```python
from build123d import *

# Parameters (mm, degrees)
SKETCH1_W           = 200
SKETCH1_H           = 70
BOSS_EXTRUDE1_DEPTH = 10
SKETCH2_W           = 200
SKETCH2_H           = 20
BOSS_EXTRUDE2_DEPTH = 30
SKETCH3_W           = 200
SKETCH3_H           = 20
BOSS_EXTRUDE3_DEPTH = 30
SKETCH4_R           = 12.5
CUT_EXTRUDE1_DEPTH  = 30
SKETCH5_W           = 50
SKETCH5_H           = 50
CUT_EXTRUDE2_DEPTH  = 30


with BuildPart() as part:
    # Sketch1 → Boss-Extrude1 (new body)
    with BuildSketch(Plane(origin=(0, 0, 0), x_dir=(1, 0, 0), z_dir=(0, 1, 0))):
        with Locations((-100, 35)):
            Rectangle(SKETCH1_W, SKETCH1_H)
    extrude(amount=BOSS_EXTRUDE1_DEPTH)

    # Sketch2 → Boss-Extrude2 (add)
    with BuildSketch(Plane(origin=(0, 10, 0), x_dir=(1, 0, 0), z_dir=(0, 1, 0))):
        with Locations((-100, 60)):
            Rectangle(SKETCH2_W, SKETCH2_H)
    extrude(amount=BOSS_EXTRUDE2_DEPTH)

    # Sketch3 → Boss-Extrude3 (add)
    with BuildSketch(Plane.XZ):
        with Locations((-100, -60)):
            Rectangle(SKETCH3_W, SKETCH3_H)
    extrude(amount=BOSS_EXTRUDE3_DEPTH)

    # Sketch4 → Cut-Extrude1 (cut)
    with BuildSketch(Plane(origin=(0, 10, 0), x_dir=(1, 0, 0), z_dir=(0, 1, 0))):
        with Locations(Location((-25, 25, 0), (0, 0, 270))):
            Circle(SKETCH4_R)
        with Locations(Location((-175, 25, 0), (0, 0, 270))):
            Circle(SKETCH4_R)
    extrude(amount=-CUT_EXTRUDE1_DEPTH, mode=Mode.SUBTRACT)

    # Sketch5 → Cut-Extrude2 (cut)
    with BuildSketch(Plane(origin=(0, 10, 0), x_dir=(1, 0, 0), z_dir=(0, 1, 0))):
        with Locations((-175, 25)):
            Rectangle(SKETCH5_W, SKETCH5_H)
    extrude(amount=-CUT_EXTRUDE2_DEPTH, mode=Mode.SUBTRACT)


solid = part.part
```
Input: part model. Units: mm. Frame: model coordinates. A direction names the side the tool comes from. Coordinates: 2 decimals unless noted, no trailing zeros. Order: outer loops, then holes, each group sorted by start corner. A loop starts at its lowest first (then second) coordinate and runs counter-clockwise, first axis right, second up. Notation, with made-up numbers: (-2, 72.5) - (6, 72.5) arc R27 ccw to (6, 101.5) - close; hole circle Ø6 at (60.5, -12). An arc over 180 degrees is marked (long way). Put each result on its own line as item: value.
1. Cut plane C-C on z = -23. Return the cut outline in (x, y), then the cut area to 3 significant figures.
Report:
outline: (-150, 0) - (-37.34, 0) - (-37.34, 10) - (-150, 10) - close; (-12.66, 0) - (0, 0) - (0, 10) - (-12.66, 10) - close
area: 1,250 mm2
2. Reachability of faces 1 (the face through (-101, 5, -70)), 2 (the face through (-76, 0, -25)), 3 (the face through (-150, 5, -25)), 4 (the face through (-76, 5, 0)), 5 (the face through (-76, 10, -25)) from +Z, -Z, +X, -X, +Y, -Y: full face, straight path, thin tool, end or side. Return the list, or none.
Report:
face 1: -Z, +X, -X, +Y, -Y
face 2: +Z, +X, -X, -Y
face 3: +Z, -X, +Y, -Y
face 4: +Z, +X, -X, +Y, -Y
face 5: +Z, +X, -X, +Y
3. Cut plane D-D on z = -33.5. Return the cut outline in (x, y).
Report:
outline: (-150, 0) - (-34.17, 0) - (-34.17, 10) - (-150, 10) - close; (-15.83, 0) - (0, 0) - (0, 10) - (-15.83, 10) - close
4. Cut plane A-A on y = 7. Return the cut outline in (x, z).
Report:
outline: (-200, -70) - (0, -70) - (0, 0) - (-150, 0) - (-150, -50) - (-200, -50) - close; hole circle Ø25 at (-25, -25)
5. Cut plane B-B on x = -25. Return the cut outline in (y, z).
Report:
outline: (-30, -70) - (40, -70) - (40, -50) - (10, -50) - (10, -37.5) - (0, -37.5) - (0, -50) - (-30, -50) - close; (0, -12.5) - (10, -12.5) - (10, 0) - (0, 0) - close
6. Contact query for flat-ended pins moving along their axis: pin 1 Ø3 at (y, z) = (7, -29.5) entering from -X; pin 2 Ø4 at (x, y) = (-129, -18) entering from +Z; pin 3 Ø6 at (x, z) = (-96, -35.5) entering from +Y. Output: stop coordinate, or through.
Report:
pin 1: stops at x = -150
pin 2: stops at z = -50
pin 3: stops at y = 10
7. Line query: line 1 along X through (y, z) = (9, -25); line 2 along Z through (x, y) = (-41, -16.5); line 3 along Y through (x, z) = (-89.5, -26). Output: solid intervals per line, ascending.
Report:
line 1: x = -150 to -37.5, -12.5 to 0
line 2: z = -70 to -50
line 3: y = 0 to 10
